```python
from build123d import *

# Parameters (mm, degrees)
F0_W     = 153
F0_H     = 69
F1_DEPTH = 1.7
F2_W     = 15
F2_H     = 4.6
F2_W_2   = 8
F2_W_3   = 1.9
F2_H_2   = 8.5
F2_W_4   = 18.5
F2_H_3   = 12.6
F2_R     = 2
F2_W_5   = 6.6
F2_H_4   = 2.1
F2_R_2   = 1.7
F3_DEPTH = 1.701
F4_W     = 89.6
F4_H     = 10.55
F5_DEPTH = 1.701
F6_R     = 1.5


with BuildPart() as f1:
    # F0 (on Top) → F1 (new body)
    with BuildSketch(Plane.XY):
        Rectangle(F0_W, F0_H)
    extrude(amount=F1_DEPTH)

    # F2 (on face) → F3 (cut, through all)
    with BuildSketch(Plane.XY.offset(1.7)):
        with Locations((-69, -32.2)):
            Rectangle(F2_W, F2_H)
        Polygon((-61.5, -29.9), (-61.5, -34.5), (-43.1, -34.5), (-43.1, -29.9), (-43.1, -21.9), (-61.5, -21.9), align=None)
        with Locations((-39.1, -32.2)):
            Rectangle(F2_W_2, F2_H)
        Polygon((-35.1, -29.9), (-35.1, -34.5), (-31.6, -34.5), (-31.6, -21.9), (-35.1, -21.9), align=None)
        with Locations((-19.35, -30.25)):
            Rectangle(F2_W_3, F2_H_2)
        with Locations((67.25, -28.2)):
            Rectangle(F2_W_4, F2_H_3)
        with Locations((-69, -24.9)):
            Circle(F2_R)
        with Locations((-69, 19.1)):
            Circle(F2_R)
        with Locations((61.5, 29.05)):
            Rectangle(F2_W_5, F2_H_4)
        with Locations((61.5, 8.55)):
            Rectangle(F2_W_5, F2_H_4)
        with Locations((-48.5, 18.8)):
            Circle(F2_R_2)
        with Locations((-18.5, 18.8)):
            Circle(F2_R_2)
        with Locations((1.5, 18.8)):
            Circle(F2_R_2)
        with Locations((-39.9, 18.8)):
            Circle(F2_R_2)
        with Locations((-9.9, 18.8)):
            Circle(F2_R_2)
        with Locations((10.1, 18.8)):
            Circle(F2_R_2)
        with Locations((70.1, 8.55)):
            Rectangle(F2_W_5, F2_H_4)
        with Locations((70.1, 29.05)):
            Rectangle(F2_W_5, F2_H_4)
        with Locations((70.1, -16.45)):
            Rectangle(F2_W_5, F2_H_4)
        with Locations((61.5, 4.05)):
            Rectangle(F2_W_5, F2_H_4)
        with Locations((70.1, 4.05)):
            Rectangle(F2_W_5, F2_H_4)
        with Locations((61.5, -16.45)):
            Rectangle(F2_W_5, F2_H_4)
        with Locations((1.5, -6.2)):
            Circle(F2_R_2)
        with Locations((-18.5, -6.2)):
            Circle(F2_R_2)
        with Locations((-9.9, -6.2)):
            Circle(F2_R_2)
        with Locations((10.1, -6.2)):
            Circle(F2_R_2)
        with Locations((-39.9, -6.2)):
            Circle(F2_R_2)
        with Locations((-48.5, -6.2)):
            Circle(F2_R_2)
    extrude(amount=-F3_DEPTH, mode=Mode.SUBTRACT)

    # F4 (on Top) → F5 (cut, through all)
    with BuildSketch(Plane.XY):
        with Locations((13.2, -29.225)):
            Rectangle(F4_W, F4_H)
    extrude(amount=F5_DEPTH, mode=Mode.SUBTRACT)

    # F6
    f6_edges = [f1.edges().sort_by_distance(p)[0] for p in [
        (-35.1, -21.9, 0.85),
        (-31.6, -21.9, 0.85),
        (-43.1, -21.9, 0.85),
        (58, -21.9, 0.85),
        (76.5, -21.9, 0.85),
        (-35.1, -29.9, 0.85),
        (-43.1, -29.9, 0.85),
        (-76.5, -29.9, 0.85),
        (-61.5, -29.9, 0.85),
        (-61.5, -21.9, 0.85),
        (76.5, 34.5, 0.85),
        (-76.5, 34.5, 0.85),
    ]]
    fillet(f6_edges, radius=F6_R)


solid = f1.part
```
Can you work these out from the model? Positions are in its coordinate system, mm. Round coordinates to 2 decimals unless told otherwise and drop trailing zeros. Order: outer loops, then holes, each group sorted by start corner. A loop starts at its lowest first (then second) coordinate and runs counter-clockwise, first axis right, second up.
(1) We'd pull the mould along Y, two halves only. Please class faces 1 (the face through (-1, 10, 0)), 2 (the face through (2.414, 20.233, 0.862)): +Y half, -Y half, draft (parallel to the pull), parting line (faces both ways), or undercut.
Results are:
face 1: draft
face 2: undercut
(2) If we section it at A-A (x = 10.1): Please give me the cut outline in (y, z).
Results are:
outline: (-23.95, 0) - (-7.9, 0) - (-7.9, 1.7) - (-23.95, 1.7) - close; (-4.5, 0) - (17.1, 0) - (17.1, 1.7) - (-4.5, 1.7) - close; (20.5, 0) - (34.5, 0) - (34.5, 1.7) - (20.5, 1.7) - close
(3) I'm going to push flat-ended pins straight in: pin 1 (2 mm diameter, centred on x = -39.9, y = -6.2, fed in from -Z); pin 2 (4.5 mm diameter, centred on x = -48.5, y = 18.8, fed in from -Z); pin 3 (0.8 mm diameter, centred on x = -52, z = 1, fed in from -Y). Where does each tip first touch, or does it pass through?
Results are:
pin 1: passes through
pin 2: stops at z = 0
pin 3: stops at y = -21.9
(4) If I drill on L1, parallel to Y at x = 10.1, z = 1.05; L2, parallel to Y at x = -69, z = 0.4; L3, parallel to Y at x = -31, z = 0.2, over which ranges is the centre line in solid material (lowest first)?
Results are:
L1: y = -23.95 to -7.9, -4.5 to 17.1, 20.5 to 34.5
L2: y = -29.9 to -26.9, -22.9 to 17.1, 21.1 to 34.5
L3: y = -23.95 to 34.5
(5) If we section it at C-C (x = -48.5): Please give me the cut outline in (y, z).
Results are:
outline: (-21.9, 0) - (-7.9, 0) - (-7.9, 1.7) - (-21.9, 1.7) - close; (-4.5, 0) - (17.1, 0) - (17.1, 1.7) - (-4.5, 1.7) - close; (20.5, 0) - (34.5, 0) - (34.5, 1.7) - (20.5, 1.7) - close
(6) If we section it at B-B (y = -6.2): Please give me the cut outline in (x, z).
Results are:
outline: (-76.5, 0) - (-50.2, 0) - (-50.2, 1.7) - (-76.5, 1.7) - close; (-46.8, 0) - (-41.6, 0) - (-41.6, 1.7) - (-46.8, 1.7) - close; (-38.2, 0) - (-20.2, 0) - (-20.2, 1.7) - (-38.2, 1.7) - close; (-16.8, 0) - (-11.6, 0) - (-11.6, 1.7) - (-16.8, 1.7) - close; (-8.2, 0) - (-0.2, 0) - (-0.2, 1.7) - (-8.2, 1.7) - close; (3.2, 0) - (8.4, 0) - (8.4, 1.7) - (3.2, 1.7) - close; (11.8, 0) - (76.5, 0) - (76.5, 1.7) - (11.8, 1.7) - close
(7) If we section it at D-D (z = 1.3): Count the separate pieces of the cut face and the enclosed holes in it, plus the area to 3 significant figures.
Results are:
separate pieces: 1
enclosed holes: 22
area: 8,750 mm2
